Part model, mm, in its own coordinate system. A direction names the side the tool comes from. Round coordinates to 2 decimals unless told otherwise and drop trailing zeros. Write each loop counter-clockwise with the first axis right and the second up, starting at its lowest first coordinate (ties: lowest second). Pieces come first, ordered by that corner, then holes.
from build123d import *

# Parameters (mm, degrees)
SKETCH1_R           = 5.842
SKETCH1_R_2         = 4.064
BOSS_EXTRUDE1_DEPTH = 7.62
SKETCH3_R           = 4.1275
BOSS_EXTRUDE2_DEPTH = 12.192
FILLET2_R           = 1.524


with BuildPart() as part:
    # Sketch1 → Boss-Extrude1 (new body)
    with BuildSketch(Plane(origin=(0, 0, 0), x_dir=(1, 0, 0), z_dir=(0, 1, 0))):
        with Locations(Location((0, 0, 0), (0, 0, 270))):  # turned: the seam where the file's is
            Circle(SKETCH1_R)
        with Locations(Location((0, 0, 0), (0, 0, 270))):  # turned: the seam where the file's is
            Circle(SKETCH1_R_2, mode=Mode.SUBTRACT)
    extrude(amount=BOSS_EXTRUDE1_DEPTH)

    # Sketch3 → Boss-Extrude2 (add)
    with BuildSketch(Plane.XZ):
        with Locations(Location((0, 0, 0), (0, 0, 90))):  # turned: the seam where the file's is
            Circle(SKETCH3_R)
    extrude(amount=BOSS_EXTRUDE2_DEPTH)

    # Fillet2
    fillet2_edges = [part.edges().sort_by_distance(p)[0] for p in [
        (0, 0, -4.1275),
    ]]
    fillet(fillet2_edges, radius=FILLET2_R)


solid = part.part
Q1. Saw through at A-A, the plane x = 0. Write the cut outline in (y, z), and give its area (3 significant figures).
Q2. Saw through at B-B, the plane y = 1.5. Write the cut outline in (x, z), and give its area (3 significant figures).
Q3. Saw through at C-C, the plane z = 0. Write the cut outline in (x, y).
Q4. Tool access for faces 4 (the flat face through (0, 0, 0)), 5 (the cylindrical face through (2.512, -6.783, -3.275)), 6 (the flat face through (1.4, 7.62, -4)): list every direction of +Z, -Z, +X, -X, +Y, -Y with a clear straight run to the whole face (end or side of a thin tool).
Q5. Drop flat-ended pins along their axis: P1, Ø1, axis at y = -3.5, z = 3.5, coming from the -X side; P2, Ø1, axis at x = -2.5, y = -10, coming from the -Z side; P3, Ø1.5, axis at x = -1.5, z = 1, coming from the +Y side. Give the stop position or say it passes through.
Q6. Saw through at D-D, the plane y = -10.5. Write the cut outline in (x, z) (1 decimal).
Q7. Wall check: line 1 (X direction, y = 4, z = 0); line 2 (Y direction, x = 5.25, z = -2); line 3 (Y direction, x = -1.5, z = -0.25). Give the ranges that are in metal, low to high.
Q8. Two-plate mould, pull along Z, no slides. Class faces 1 (the flat face through (0, -12.192, 0)), 2 (the cylindrical face through (-3.967, 3.757, -0.881)), 3 (the cylindrical face through (-3.6, 3.8, -4.6)): released by +Z, released by -Z, zero draft, split by the parting line, or undercut.
Computed:
1. outline: (-12.19, -4.13) - (-1.52, -4.13) arc R1.52 cw to (0, -5.65) - (0, -5.84) - (7.62, -5.84) - (7.62, -4.06) - (0, -4.06) - (0, 4.06) - (7.62, 4.06) - (7.62, 5.84) - (0, 5.84) - (0, 5.65) arc R1.52 cw to (-1.52, 4.13) - (-12.19, 4.13) - close
1. area: 129 mm2
2. outline: circle Ø11.68 at (0, 0); hole circle Ø8.13 at (0, 0)
2. area: 55.3 mm2
3. outline: (-5.84, 0) - (-5.65, 0) arc R1.52 cw to (-4.13, -1.52) - (-4.13, -12.19) - (4.13, -12.19) - (4.13, -1.52) arc R1.52 cw to (5.65, 0) - (5.84, 0) - (5.84, 7.62) - (4.06, 7.62) - (4.06, 0) - (-4.06, 0) - (-4.06, 7.62) - (-5.84, 7.62) - close
4. face 4: +Y
4. face 5: -Y
4. face 6: +Z, -Z, +X, -X, +Y
5. P1: stops at x = -2.83
5. P2: stops at z = -3.61
5. P3: stops at y = 0
6. outline: circle Ø8.3 at (0, 0)
7. line 1: x = -5.84 to -4.06, 4.06 to 5.84
7. line 2: y = 0 to 7.62
7. line 3: y = -12.19 to 0
8. face 1: zero draft
8. face 2: undercut
8. face 3: split by the parting line
